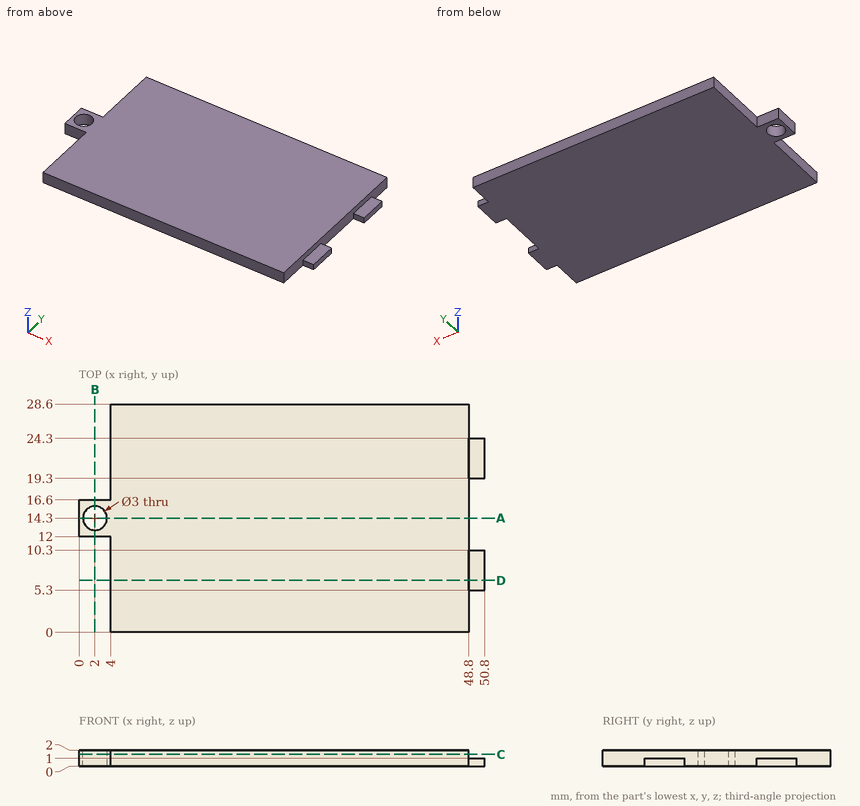
The drawing under review shows one solid part. Ordinate dimensions are in mm from its lowest x, y, z. Round coordinates to 2 decimals unless told otherwise and drop trailing zeros. Loops run counter-clockwise (first coordinate to the right, second up) from the corner with the lowest first, then second, coordinate; pieces in that order, holes last. Notation, with made-up numbers: (68.5, 1.25) -> (83.5, 1.25) arc R35 ccw to (83.5, 37.25) -> close; hole circle Ø6 at (74, -18). An arc over 180 degrees is marked (long way). One line per question, with ' | ' between items. Start each with the question number.
Item 1: For pin 1 (0.6 mm diameter, centred on y = 15, z = 0.5, fed in from +X); pin 2 (0.8 mm diameter, centred on x = 50, z = 0.5, fed in from +Y); pin 3 (2 mm diameter, centred on x = 50, y = 20.5, fed in from +Z), all flat-tipped, find the tip position at first contact; note any pin that passes through.
Item 2: Add section C-C, the plane z = 1.5. Write out the cut boundary in (x, y).
Item 3: Add section A-A, the plane y = 14.3. Write out the cut boundary in (x, z).
Item 4: Wall thickness on line 1 along Y through (x, z) = (2, 1); line 2 along X through (y, z) = (20.25, 0.45); line 3 along X through (y, z) = (11.25, 1.65): over which ranges is each line inside the solid? List them lowest first. Write a range as [from, to].
Item 5: Add section D-D, the plane y = 6.5. Write out the cut boundary in (x, z), then the cut area to 3 significant figures.
Item 6: Add section B-B, the plane x = 2. Write out the cut boundary in (y, z), then the cut area to 3 significant figures.
Return value:
1) pin 1: stops at x = 48.8 | pin 2: stops at y = 24.3 | pin 3: stops at z = 1
2) outline: (0, 12) -> (4, 12) -> (4, 0) -> (48.8, 0) -> (48.8, 28.6) -> (4, 28.6) -> (4, 16.6) -> (0, 16.6) -> close; hole circle Ø3 at (2, 14.3)
3) outline: (0, 0) -> (0.5, 0) -> (0.5, 2) -> (0, 2) -> close; (3.5, 0) -> (48.8, 0) -> (48.8, 2) -> (3.5, 2) -> close
4) line 1: y = [12, 12.8], [15.8, 16.6] | line 2: x = [4, 50.8] | line 3: x = [4, 48.8]
5) outline: (4, 0) -> (50.8, 0) -> (50.8, 1) -> (48.8, 1) -> (48.8, 2) -> (4, 2) -> close | area: 91.6 mm2
6) outline: (12, 0) -> (12.8, 0) -> (12.8, 2) -> (12, 2) -> close; (15.8, 0) -> (16.6, 0) -> (16.6, 2) -> (15.8, 2) -> close | area: 3.20 mm2
